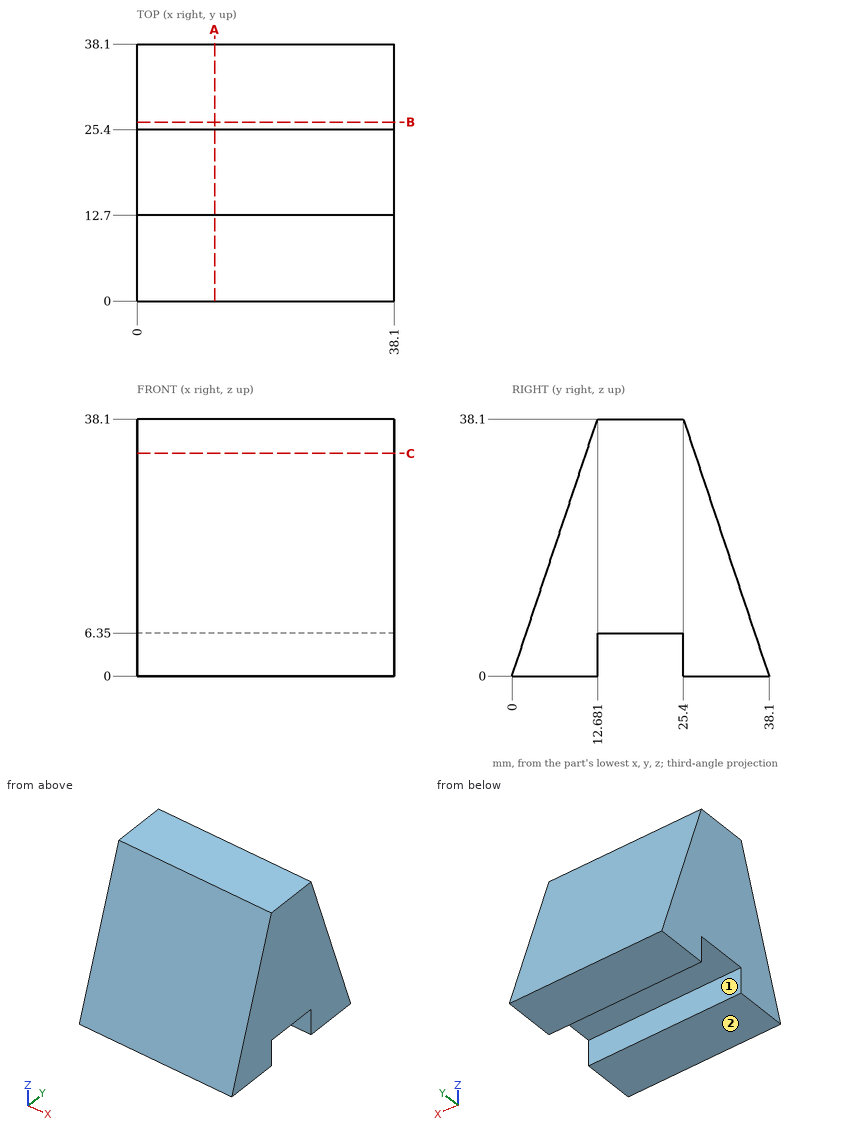
Answer from the drawing. Dimensions are ordinates in mm from the lowest x, y and z of the part. A direction names the side the tool comes from. Give positions to 0.01 mm unless a question says otherwise; leave off trailing zeros. Order: outer loops, then holes, each group sorted by start corner. A loop starts at its lowest first (then second) coordinate and runs counter-clockwise, first axis right, second up. Notation, with made-up numbers: (31, 65) - (39, 65) arc R12 ccw to (39, 88) - close; hole circle Ø11 at (85.5, 46.5). An arc over 180 degrees is marked (long way). One line per item, written item: value. Start each with the question number.
1) Find the intervals of material crossed by L1, parallel to Z at x = 5.5, y = 15; L2, parallel to Y at x = 33, z = 4.5; L3, parallel to Y at x = 29, z = 34.5, in increasing order.
2) A cutting plane is placed at C-C on z = 33. Give the vertices of the cut face in (x, y).
3) A tool of negligible diameter and unlimited length cuts with its end or side. For the marked faces 1 and 2, from which of +Z, -Z, +X, -X, +Y, -Y can it reach the whole face along a straight path? Write none if from no direction.
4) Given pin 1 Ø1.5 at (x, y) = (31.5, 33) entering from -Z; pin 2 Ø1 at (x, z) = (7.5, 27.5) entering from -Y; pin 3 Ø3 at (x, z) = (28.5, 18.5) entering from -Y; pin 4 Ø2 at (x, z) = (9, 23.5) entering from -Y, each flat-ended and moving along its own axis, determine where each tip first touches the part or whether it passes through.
5) A cutting plane is placed at B-B on y = 26.5. Give the vertices of the cut face in (x, z).
6) A cutting plane is placed at A-A on x = 11.5. Give the vertices of the cut face in (y, z).
Answer sheet:
1. L1: z = 6.35 to 38.1
1. L2: y = 1.5 to 12.7, 25.4 to 36.6
1. L3: y = 11.48 to 26.6
2. outline: (0, 10.98) - (38.1, 10.98) - (38.1, 27.1) - (0, 27.1) - close
3. face 1: -Z, +X, -X
3. face 2: -Z, +X, -X, +Y, -Y
4. pin 1: stops at z = 0
4. pin 2: stops at y = 8.99
4. pin 3: stops at y = 5.66
4. pin 4: stops at y = 7.49
5. outline: (0, 0) - (38.1, 0) - (38.1, 34.8) - (0, 34.8) - close
6. outline: (0, 0) - (12.7, 0) - (12.7, 6.35) - (25.4, 6.35) - (25.4, 0) - (38.1, 0) - (25.4, 38.1) - (12.68, 38.1) - close
